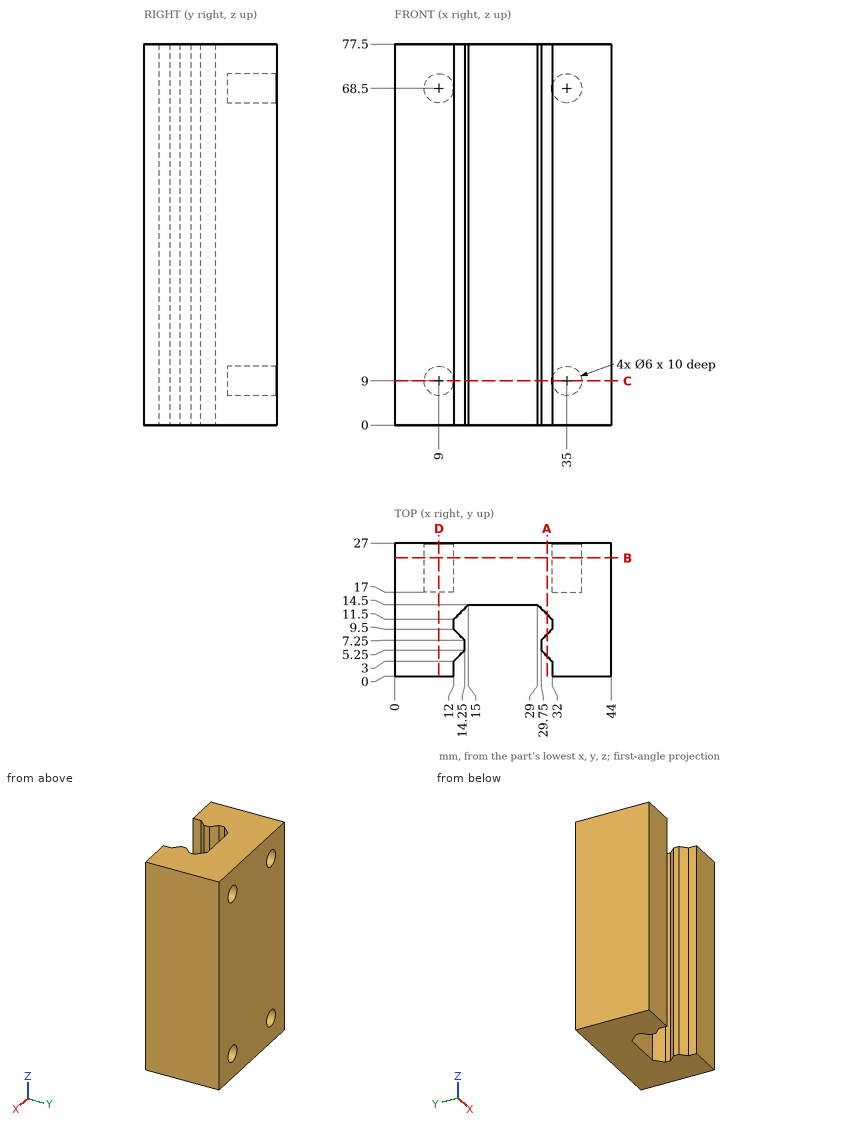
Print and shaded views of the part. All mm, measured from the part's lowest x, y and z. Round coordinates to 2 decimals unless told otherwise and drop trailing zeros. Write each loop counter-clockwise with the first axis right and the second up, starting at its lowest first coordinate (ties: lowest second). Pieces come first, ordered by that corner, then holes. Notation, with made-up numbers: (-36, 79.25) - (-28, 79.25) arc R17 cw to (-28, 111.25) - close; hole circle Ø6 at (62, 47.25). An arc over 180 degrees is marked (long way). Write each question's results on one line, items separated by ' | '. Start each with the question number.
Item 1: Saw through at B-B (y = 24). Write the cut outline in (x, z), and give its area (3 significant figures).
Item 2: Drop flat-ended pins along their axis: P1, Ø3, axis at x = 35, z = 68, coming from the +Y side; P2, Ø4, axis at x = 22, z = 48, coming from the -Y side. Give the stop position or say it passes through.
Item 3: Wall check: L1, parallel to X at y = 20.25, z = 68.5; L2, parallel to Z at x = 35, y = 20.5; L3, parallel to X at y = 17.25, z = 11. Give the ranges that are in metal, low to high. Write a range as [from, to].
Item 4: Saw through at D-D (x = 9). Write the cut outline in (y, z).
Item 5: Saw through at A-A (x = 31). Write the cut outline in (y, z).
Item 6: Saw through at C-C (z = 9). Write the cut outline in (x, y).
Results are:
1) outline: (0, 0) - (44, 0) - (44, 77.5) - (0, 77.5) - close; hole circle Ø6 at (9, 9); hole circle Ø6 at (9, 68.5); hole circle Ø6 at (35, 9); hole circle Ø6 at (35, 68.5) | area: 3,300 mm²
2) P1: stops at y = 17 | P2: stops at y = 14.5
3) L1: x = [0, 6], [12, 32], [38, 44] | L2: z = [0, 6], [12, 65.5], [71.5, 77.5] | L3: x = [0, 6.76], [11.24, 32.76], [37.24, 44]
4) outline: (0, 0) - (27, 0) - (27, 6) - (17, 6) - (17, 12) - (27, 12) - (27, 65.5) - (17, 65.5) - (17, 71.5) - (27, 71.5) - (27, 77.5) - (0, 77.5) - close
5) outline: (4, 0) - (8.5, 0) - (8.5, 77.5) - (4, 77.5) - close; (12.5, 0) - (27, 0) - (27, 77.5) - (12.5, 77.5) - close
6) outline: (0, 0) - (12, 0) - (12, 3) - (14.25, 5.25) - (14.25, 7.25) - (12, 9.5) - (12, 11.5) - (15, 14.5) - (29, 14.5) - (32, 11.5) - (32, 9.5) - (29.75, 7.25) - (29.75, 5.25) - (32, 3) - (32, 0) - (44, 0) - (44, 27) - (38, 27) - (38, 17) - (32, 17) - (32, 27) - (12, 27) - (12, 17) - (6, 17) - (6, 27) - (0, 27) - close
